Check sheet for the modelled part. Datum: model origin and axes. Units: mm. A direction names the side the tool comes from. Give positions to 0.01 mm unless a question says otherwise; leave off trailing zeros. Loops run counter-clockwise (first coordinate to the right, second up) from the corner with the lowest first, then second, coordinate; pieces in that order, holes last. Notation, with made-up numbers: (9, 13.25) - (20, 13.25) arc R26 cw to (20, 42.25) - close; hole circle Ø10 at (-18.75, 72). An arc over 180 degrees is marked (long way). Use CSV: the item, a comma, the result in double quotes.
Autodesk Inventor part; units mm, degrees
ref_plane "YZ Plane" through (0, 0, 0) normal (1, 0, 0) x (0, 1, 0)
ref_plane "XZ Plane" through (0, 0, 0) normal (0, 1, 0) x (-1, 0, 0)
ref_plane "XY Plane" through (0, 0, 0) normal (0, 0, 1) x (1, 0, 0)
sketch "Sketch1" plane through (0, 0, 0) normal (0, 0, 1) x (1, 0, 0)
  arc A0 (-210.4144, 46.4953) -> (-210.4144, -19.5447) centre (-210.4144, 13.4753) ccw
  arc A1 (-15.5964, -19.5447) -> (-15.5964, 46.4953) centre (-15.5964, 13.4753) ccw
  line L0 (-210.4144, 46.4953) -> (-15.5964, 46.4953)
  line L1 (-210.4144, -19.5447) -> (-15.5964, -19.5447)
  arc A2 (-15.5964, -23.3547) -> (-15.5964, 50.3053) centre (-15.5964, 13.4753) ccw
  line L2 (-15.5964, -23.3547) -> (-210.4144, -23.3547)
  arc A3 (-210.4144, 50.3053) -> (-210.4144, -23.3547) centre (-210.4144, 13.4753) ccw
  line L3 (-210.4144, 50.3053) -> (-15.5964, 50.3053)
  point P0 (0, 0)
  dimension "d0" = 66.04
  dimension "d1" = 66.04
  dimension "d2" = 194.818
  dimension "d3" = 3.81
extrude "Extrusion1" add sketch "Sketch1" along normal blind 17.78
properties part number "Chassis_7.67inBelt"
1. Release check for a two-part mould opening along Y. For faces 1 (the face through (-112, -23.355, 9)), 2 (the face through (21.225, 14.285, 8.766)), 3 (the face through (-243.426, 12.749, 8.766)) record: released by +Y, released by -Y, zero draft, split by the parting line, or undercut.
Completed:
face 1,"released by -Y"
face 2,"split by the parting line"
face 3,"undercut"
2. Sectioned sample at C-C, the plane z = 14.25. Record the boundary of the cut face in (x, y).
Completed:
outline,"(-210.41, -23.35) - (-15.6, -23.35) arc R36.83 ccw to (-15.6, 50.31) - (-210.41, 50.31) arc R36.83 ccw to start; hole (-210.41, -19.54) - (-15.6, -19.54) arc R33.02 ccw to (-15.6, 46.5) - (-210.41, 46.5) arc R33.02 ccw to start"
3. Scan lines: line 1 along X through (y, z) = (13, 10.25); line 2 along Y through (x, z) = (-140, 3); line 3 along X through (y, z) = (20, 7.75). Record each from-to range of solid material in increasing order.
Completed:
line 1,"x = -247.24 to -243.43, 17.42 to 21.23"
line 2,"y = -23.35 to -19.54, 46.5 to 50.31"
line 3,"x = -246.66 to -242.78, 16.77 to 20.65"
4. Go/stop test with flat-tipped pins: pin 1 Ø2 at (y, z) = (4, 12.5) entering from -X; pin 2 Ø8 at (y, z) = (33, 2.5) entering from +X; pin 3 Ø5 at (x, y) = (-168.5, 42.5) entering from -Z; pin 4 Ø4 at (y, z) = (25, 7) entering from -X. Record where each tip stops, or that it passes through.
Completed:
pin 1,"stops at x = -246.26"
pin 2,"stops at x = 17.8"
pin 3,"passes through"
pin 4,"stops at x = -245.99"
5. Set-up check for faces 4 (the face through (-114, 46.495, 9)), 5 (the face through (-114, -22, 0)): record each of +Z, -Z, +X, -X, +Y, -Y from which the full face is reachable in a straight line by a thin tool's end or side.
Completed:
face 4,"+Z, -Z"
face 5,"-Z, +X, -X, +Y, -Y"
6. Sectioned sample at A-A, the plane x = -187. Record the boundary of the cut face in (y, z), and give its area (3 significant figures).
Completed:
outline,"(-23.35, 0) - (-19.54, 0) - (-19.54, 17.78) - (-23.35, 17.78) - close; (46.5, 0) - (50.31, 0) - (50.31, 17.78) - (46.5, 17.78) - close"
area,"135 mm²"
7. Sectioned sample at B-B, the plane y = 20.5. Record the boundary of the cut face in (x, z).
Completed:
outline,"(-246.57, 0) - (-242.68, 0) - (-242.68, 17.78) - (-246.57, 17.78) - close; (16.67, 0) - (20.56, 0) - (20.56, 17.78) - (16.67, 17.78) - close"
